Verification items for the finished model (mm, model axes). Round coordinates to 2 decimals unless told otherwise and drop trailing zeros. Write each loop counter-clockwise with the first axis right and the second up, starting at its lowest first coordinate (ties: lowest second). Pieces come first, ordered by that corner, then holes. Notation, with made-up numbers: (15.5, 29.5) - (63.5, 29.5) arc R31 ccw to (63.5, 55.5) - close; hole circle Ø2 at (10, -23.75). An arc over 180 degrees is marked (long way). Answer as a JSON object with one key per item and string values. Group by question number.
1) Section check A-A (z = 22). Enter the section's corners in (x, y).
2) Go/stop test with flat-tipped pins: pin 1 Ø1 at (x, z) = (10, -15) entering from -Y; pin 2 Ø3 at (y, z) = (7.5, -1) entering from -X; pin 3 Ø6 at (x, z) = (-16.5, 18.5) entering from -Y. Record where each tip stops, or that it passes through.
3) Thickness scan on line 1 (Y direction, x = -15, z = 27); line 2 (Y direction, x = 11, z = 17); line 3 (X direction, y = 6, z = -6). Record the ranges inside material, lowest first.
```python
from build123d import *

# Parameters (mm, degrees)
BOSS_EXTRUDE1_DEPTH = 10
CUT_EXTRUDE1_DEPTH  = 58.879184514
CUT_EXTRUDE2_DEPTH  = 75.204110398
FILLET1_R           = 2.5


with BuildPart() as part:
    # Sketch1 → Boss-Extrude1 (new body)
    with BuildSketch(Plane(origin=(0, 0, 0), x_dir=(1, 0, 0), z_dir=(0, 1, 0))):
        Polygon((-22.5, -15), (22.5, 35), (22.5, -35), (-22.5, -35), align=None)
    extrude(amount=BOSS_EXTRUDE1_DEPTH)

    # Sketch2 → Cut-Extrude1 (cut, through all)
    with BuildSketch(Plane(origin=(22.5, 0, 0), x_dir=(0, 0, -1), z_dir=(1, 0, 0))):
        Polygon((35, 0), (35, 5), (-15, 0), align=None)
        Polygon((35, 10), (-15, 10), (35, 5), align=None)
    extrude(amount=-CUT_EXTRUDE1_DEPTH, mode=Mode.SUBTRACT)

    # Sketch3 → Cut-Extrude2 (cut, through all)
    with BuildSketch(Plane.XY.offset(35)):
        Polygon((-22.5, 10), (-22.5, 5), (22.5, 10), align=None)
        Polygon((-22.5, 0), (22.5, 0), (-22.5, 5), align=None)
    extrude(amount=-CUT_EXTRUDE2_DEPTH, mode=Mode.SUBTRACT)

    # Fillet1
    # the kernel refuses this fillet: 2.5 mm, written as the material it takes off along each edge
    with BuildSketch(Plane(origin=(-3.900636109, 2.066595988, -5.665959879), x_dir=(-0.049586965018551935, 0.9972489631508745, 0.0550966277983907), z_dir=(0.667124384994991, 0.07412493166611012, -0.7412493166611013)), Plane(origin=(26.400636109, 4.566595988, -39.334040121), x_dir=(-0.04958696501855178, -0.9972489631508747, 0.05509662779839086), z_dir=(-0.667124384994991, 0.07412493166611012, 0.7412493166611013))) as fillet1_piece_1:
        with BuildLine():
            CenterArc((FILLET1_R * 0.935510365796, FILLET1_R), FILLET1_R, 183.816685755, 86.183314245)
            Line((-FILLET1_R * 0.0622717598086, FILLET1_R * 0.93343552131), (0, 0))
            Line((0, 0), (FILLET1_R * 0.935510365796, 0))
        make_face()
    extrude(amount=45.420723481, mode=Mode.SUBTRACT)
    with BuildSketch(Plane(origin=(3.840238573, 7.926693175, -14.266931748), x_dir=(0.04958696501855149, -0.9972489631508746, -0.05509662779839123), z_dir=(-0.6671243849949912, -0.07412493166611021, 0.7412493166611013)), Plane(origin=(-26.340238573, 5.426693175, 19.266931748), x_dir=(0.04958696501855112, 0.9972489631508746, -0.05509662779839134), z_dir=(0.6671243849949912, -0.07412493166611005, -0.7412493166611013))) as fillet1_piece_2:
        with BuildLine():
            CenterArc((FILLET1_R * 0.921024902586, FILLET1_R), FILLET1_R, 184.708312873, 85.291687127)
            Line((-FILLET1_R * 0.0756005855297, FILLET1_R * 0.917916893107), (0, 0))
            Line((0, 0), (FILLET1_R * 0.921024902586, 0))
        make_face()
    extrude(amount=45.23965519, mode=Mode.SUBTRACT)


solid = part.part
```
Returned:
{
 "1": {"outline": "(-22.5, 5) - (22.5, 0) - (22.5, 10) - close"},
 "2": {"pin 1": "y = 2.95", "pin 2": "x = -7.57", "pin 3": "y = 4"},
 "3": {"line 1": "4.17 to 5.83", "line 2": "1.28 to 8.72", "line 3": "-3.2 to 22.5"}
}
